```python
from build123d import *

# Parameters (mm, degrees)
EXTRUDE_1_DEPTH     = 20
SKETCH_3_R          = 2
CUT_EXTRUDE_1_DEPTH = 3
CHAMFER_1_SIZE      = 2


with BuildPart() as part:
    # 草图1 → 凸台-拉伸1 (new body)
    with BuildSketch(Plane(origin=(0, 0, 0), x_dir=(1, 0, 0), z_dir=(0, 1, 0))):
        with BuildLine():
            Line((0, 15), (95, 15))
            ThreePointArc((95, 15), (110, 0), (95, -15))
            Line((95, -15), (0, -15))
            ThreePointArc((0, -15), (-15, 0), (0, 15))
        make_face()
    extrude(amount=EXTRUDE_1_DEPTH)

    # 草图3 → 切除-拉伸1 (cut)
    with BuildSketch(Plane(origin=(0, 20, 0), x_dir=(1, 0, 0), z_dir=(0, 1, 0))):
        with Locations(Location((0, 0, 0), (0, 0, 270))):
            Circle(SKETCH_3_R)
        with Locations(Location((95, 0, 0), (0, 0, 270))):
            Circle(SKETCH_3_R)
    extrude(amount=-CUT_EXTRUDE_1_DEPTH, mode=Mode.SUBTRACT)

    # 倒角1
    chamfer_1_edges = [part.edges().sort_by_distance(p)[0] for p in [
        (47.5, 0, -15),
        (110, 0, 0),
        (47.5, 0, 15),
        (-15, 0, 0),
    ]]
    chamfer(chamfer_1_edges, length=CHAMFER_1_SIZE)


solid = part.part
```
Work out the finished part from the listing and answer in its coordinate system (mm). A direction names the side the tool comes from. Round coordinates to 2 decimals unless told otherwise and drop trailing zeros. Loops run counter-clockwise (first coordinate to the right, second up) from the corner with the lowest first, then second, coordinate; pieces in that order, holes last. Notation, with made-up numbers: (-10, 48) -> (-4, 48) arc R33 ccw to (-4, 82) -> close; hole circle Ø6 at (49.25, 62). An arc over 180 degrees is marked (long way). Write each question's results on one line, items separated by ' | '. Start each with the question number.
1. A tool of negligible diameter and unlimited length cuts with its end or side. For faces 1 (the face through (0, 17, 0)), 2 (the face through (48, 20, 0)), from which of +Z, -Z, +X, -X, +Y, -Y can it reach the whole face along a straight path? Write none if from no direction.
2. Given pin 1 Ø3 at (x, z) = (95.5, 0.5) entering from +Y; pin 2 Ø3 at (x, y) = (-2, 18) entering from +Z; pin 3 Ø4 at (y, z) = (17.5, 5.5) entering from +X; pin 4 Ø2.5 at (x, z) = (95, 0) entering from +Y, each flat-ended and moving along its own axis, determine where each tip first touches the part or whether it passes through.
3. For a pull along X with two mould halves and no side action, classify faces 3 (the face through (97, 19, 0)), 4 (the face through (48, 11, 15)), 5 (the face through (-15, 11, 0)) as +X half, -X half, draft (parallel to the pull), parting line (faces both ways), or undercut.
4. Find the intervals of material crossed by probe 1 along X at (y, z) = (18.3, 0); probe 2 along X at (y, z) = (4.5, 13); probe 3 along X at (y, z) = (12.5, -9), in increasing order. Write a range as from..to.
5. Section A-A (y = 5) is taken. Determine the outline of the cut face in (x, z), plus the area to 3 significant figures.
Evaluation:
1) face 1: +Y | face 2: +Z, -Z, +X, -X, +Y
2) pin 1: stops at y = 20 | pin 2: stops at z = 14.99 | pin 3: stops at x = 109.59 | pin 4: stops at y = 17
3) face 3: undercut | face 4: draft | face 5: -X half
4) probe 1: x = -15..-2, 2..93, 97..110 | probe 2: x = -7.48..102.48 | probe 3: x = -12..107
5) outline: (0, -15) -> (95, -15) arc R15 ccw to (95, 15) -> (0, 15) arc R15 ccw to start | area: 3,560 mm2
